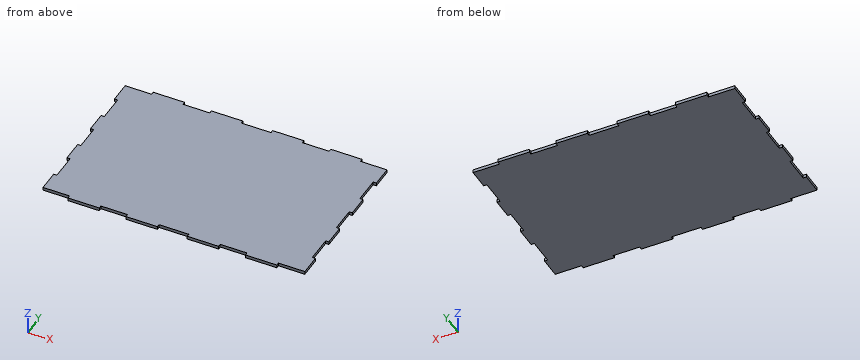
from build123d import *

# Parameters (mm, degrees)
F1_DEPTH = 3


with BuildPart() as f1:
    # F0 (on Top) → F1 (new body)
    with BuildSketch(Plane.XY):
        Polygon((-99.75, -77), (-99.75, -80), (-84.75, -80), (-69.75, -80), (-69.75, -77), (-44.25, -77), (-44.25, -80), (-29.25, -80), (-14.25, -80), (-14.25, -77), (14.25, -77), (14.25, -80), (44.25, -80), (44.25, -77), (69.75, -77), (69.75, -80), (99.75, -80), (99.75, -77), (125, -77), (125, -57), (122, -57), (122, -32), (125, -32), (125, -12), (122, -12), (122, 12), (123.5, 22), (122, 32), (122, 57), (125, 57), (125, 77), (99.75, 77), (99.75, 80), (69.75, 80), (69.75, 77), (44.25, 77), (44.25, 80), (14.25, 80), (14.25, 77), (-14.25, 77), (-14.25, 80), (-44.25, 80), (-44.25, 77), (-69.75, 77), (-69.75, 80), (-99.75, 80), (-99.75, 77), (-125, 77), (-125, 57), (-122, 57), (-122, 32), (-125, 32), (-125, 12), (-122, 12), (-122, -12), (-125, -12), (-125, -32), (-122, -32), (-122, -57), (-125, -57), (-125, -77), align=None)
        Polygon((123.5, 22), (122, 12), (125, 12), align=None)
        Polygon((123.5, 22), (125, 12), (125, 22), align=None)
        Polygon((122, 32), (123.5, 22), (125, 32), align=None)
        Polygon((125, 32), (123.5, 22), (125, 22), align=None)
    extrude(amount=F1_DEPTH)


solid = f1.part
Source: CAD feature listing. Evaluate the final solid. Frame: model axes, mm. Coordinates: 2 decimals unless noted, no trailing zeros. Order: outer loops, then holes, each group sorted by start corner. A loop starts at its lowest first (then second) coordinate and runs counter-clockwise, first axis right, second up. Notation, with made-up numbers: M 66.25,80 L 111.25,80 A14 ccw 111.25,99 Z; hole C 10,21.25 d3. An arc over 180 degrees is marked long. Write each question's results on one line, items separated by ' | '. Start each with the question number.
Item 1: Cut plane A-A (y = 42.5). Return loops of the section in (x, z), and give its area (3 significant figures).
Item 2: Line query: probe 1 along Y at (x, z) = (-108, 0.7); probe 2 along X at (y, z) = (-50, 0.75). Output: solid intervals per line, ascending.
Item 3: First-contact query: pin 1 Ø1.5 at (x, z) = (-124, 2) entering from -Y; pin 2 Ø0.9 at (y, z) = (78, 2) entering from +X; pin 3 Ø1.5 at (y, z) = (-2.5, 1.5) entering from +X. Flat tips, straight axial feed; report the tip coordinate or a pass-through.
Item 4: Cut plane B-B (x = -105.5). Return loops of the section in (y, z), and give its area (3 significant figures).
Checked values:
1) outline: M -122,0 L 122,0 L 122,3 L -122,3 Z | area: 732 mm2
2) probe 1: y = -77 to 77 | probe 2: x = -122 to 122
3) pin 1: stops at y = -77 | pin 2: stops at x = 99.75 | pin 3: stops at x = 122
4) outline: M -77,0 L 77,0 L 77,3 L -77,3 Z | area: 462 mm2
